Design review of the part built by this model. Coordinates are the model's own, in mm. Face numbers are marked on the shaded views. A direction names the side the tool comes from. Coordinates: 2 decimals unless noted, no trailing zeros. Loops run counter-clockwise (first coordinate to the right, second up) from the corner with the lowest first, then second, coordinate; pieces in that order, holes last. Notation, with made-up numbers: M -40,-17 L 12,-17 A27 ccw 12,15 Z; hole C 33.25,50.5 d11. An arc over 180 degrees is marked long. Put each result on its own line as item: value. Start each with the question number.
(1) Take a section at D-D, the plane x = -47. Give the boundary of the cut face in (y, z), then the cut area to 3 significant figures.
(2) For probe 1 along Z at (x, y) = (27.5, 11); probe 2 along Y at (x, z) = (24.5, -33.5); probe 3 along Z at (x, y) = (61.5, 15.5), list the stretches that pass through material, from the lowest coordinate up. Write a range as [from, to].
(3) Clearance check with flat-ended pins moving along their axes: pin 1 (2 mm diameter, centred on y = 16.5, z = -2, fed in from -X); pin 2 (1.5 mm diameter, centred on x = -29, z = 4.5, fed in from +Y); pin 3 (1 mm diameter, centred on x = -27, y = 12.5, fed in from -Z); pin 4 (10 mm diameter, centred on y = 17, z = 2, fed in from +X). State where each tip first meets the part, or that it passes through.
(4) The part is to be moulded in two halves that separate along Z. For the marked faces 1, 2, 3 and 4, say which applies: +Z half, -Z half, draft (parallel to the pull), parting line (faces both ways), or undercut.
(5) For the marked faces 5 and 6, list the 3-axis set-ups (+Z, -Z, +X, -X, +Y, -Y) from which the entire face can be reached by the end or side of a thin tool; tool diameter is ignored.
(6) Take a section at A-A, the plane y = 14. Give the boundary of the cut face in (x, z), then the cut area to 3 significant figures.
(7) Take a section at C-C, the plane z = 30.5. Give the boundary of the cut face in (x, y).
(8) Take a section at B-B, the plane x = 27. Give the boundary of the cut face in (y, z), then the cut area to 3 significant figures.
```python
from build123d import *

# Parameters (mm, degrees)
BOSS_EXTRUDE1_DEPTH = 25.4
BOSS_EXTRUDE2_START = -30.48
BOSS_EXTRUDE2_DEPTH = 5.08
SKETCH4_R           = 1.7018
BOSS_EXTRUDE3_DEPTH = 20.4964
BOSS_EXTRUDE4_START = -6.35
BOSS_EXTRUDE4_DEPTH = 6.35


with BuildPart() as part:
    # Sketch1 → Boss-Extrude1 (new body)
    with BuildSketch(Plane(origin=(0, 0, 0), x_dir=(1, 0, 0), z_dir=(0, 1, 0))):
        with BuildLine():
            Line((0, 43.18), (35.56, 43.18))
            ThreePointArc((35.56, 43.18), (78.74, 0), (35.56, -43.18))
            Line((35.56, -43.18), (0, -43.18))
            ThreePointArc((0, -43.18), (-43.18, 0), (0, 43.18))
        make_face()
        with BuildLine():
            Line((0, 40.64), (35.56, 40.64))
            ThreePointArc((35.56, 40.64), (76.2, 0), (35.56, -40.64))
            Line((35.56, -40.64), (0, -40.64))
            ThreePointArc((0, -40.64), (-40.64, 0), (0, 40.64))
        make_face(mode=Mode.SUBTRACT)
    extrude(amount=BOSS_EXTRUDE1_DEPTH)

    # Sketch3 → Boss-Extrude2 (add)
    with BuildSketch(Plane(origin=(0, 25.4, 0), x_dir=(1, 0, 0), z_dir=(0, 1, 0)).offset(BOSS_EXTRUDE2_START)):
        with BuildLine():
            Line((0, 43.18), (35.56, 43.18))
            ThreePointArc((35.56, 43.18), (78.74, 0), (35.56, -43.18))
            Line((35.56, -43.18), (0, -43.18))
            ThreePointArc((0, -43.18), (-43.18, 0), (0, 43.18))
        make_face()
    extrude(amount=BOSS_EXTRUDE2_DEPTH)

    # Sketch4 → Boss-Extrude3 (add)
    with BuildSketch(Plane(origin=(0, 0, 0), x_dir=(1, 0, 0), z_dir=(0, 1, 0))):
        with Locations(Location((43.18, 0, 0), (0, 0, 270))):
            Circle(SKETCH4_R)
        with Locations(Location((-7.62, 0, 0), (0, 0, 270))):
            Circle(SKETCH4_R)
    extrude(amount=BOSS_EXTRUDE3_DEPTH)

    # Sketch5 → Boss-Extrude4 (add)
    with BuildSketch(Plane(origin=(0, 25.4, 0), x_dir=(1, 0, 0), z_dir=(0, 1, 0)).offset(BOSS_EXTRUDE4_START)):
        with BuildLine():
            Line((-40.416376905, 4.257473181), (-78.516376905, 4.257473181))
            Line((-78.516376905, 4.257473181), (-78.516376905, -4.307631169))
            Line((-78.516376905, -4.307631169), (-40.411061774, -4.307631169))
            ThreePointArc((-40.411061774, -4.307631169), (-40.639992175, -0.025219409), (-40.416376905, 4.257473181))
        make_face()
        with BuildLine():
            Line((75.777132348, 5.847381095), (113.877132348, 5.847381095))
            Line((113.877132348, 5.847381095), (113.877132348, -5.847381095))
            Line((113.877132348, -5.847381095), (75.777132348, -5.847381095))
            ThreePointArc((75.777132348, -5.847381095), (76.2, 0), (75.777132348, 5.847381095))
        make_face()
    extrude(amount=BOSS_EXTRUDE4_DEPTH)


solid = part.part
```
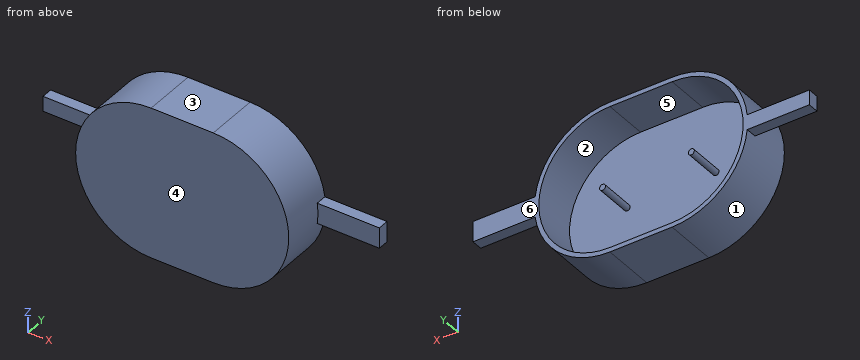
Computed values:
1. outline: M 19.05,-4.26 L 25.4,-4.26 L 25.4,4.31 L 19.05,4.31 Z
1. area: 54.4 mm^2
2. probe 1: z = [-43.18, -40.64], [40.64, 43.18]
2. probe 2: y = [-5.08, 0]
2. probe 3: z = [-34.52, -31.28], [31.28, 34.52]
3. pin 1: stops at x = -43.17
3. pin 2: stops at y = 0
3. pin 3: stops at z = -34.09
3. pin 4: stops at x = 113.88
4. face 1: parting line
4. face 2: undercut
4. face 3: +Z half
4. face 4: draft
5. face 5: +Y
5. face 6: +Z, -Z, +X, -X, +Y
6. outline: C -7.62,0 d3.4; M 0,-43.18 L 35.56,-43.18 A43.18 ccw 35.56,43.18 L 0,43.18 A43.18 ccw Z; C 43.18,0 d3.4; hole M 0,-40.64 L 35.56,-40.64 A40.64 ccw 35.56,40.64 L 0,40.64 A40.64 ccw Z
6. area: 868 mm^2
7. outline: M -30.57,-5.08 L 66.13,-5.08 L 66.13,25.4 L 62.42,25.4 L 62.42,0 L -26.86,0 L -26.86,25.4 L -30.57,25.4 Z
8. outline: M -5.08,-43.18 L 25.4,-43.18 L 25.4,-40.64 L 0,-40.64 L 0,40.64 L 25.4,40.64 L 25.4,43.18 L -5.08,43.18 Z
8. area: 568 mm^2
